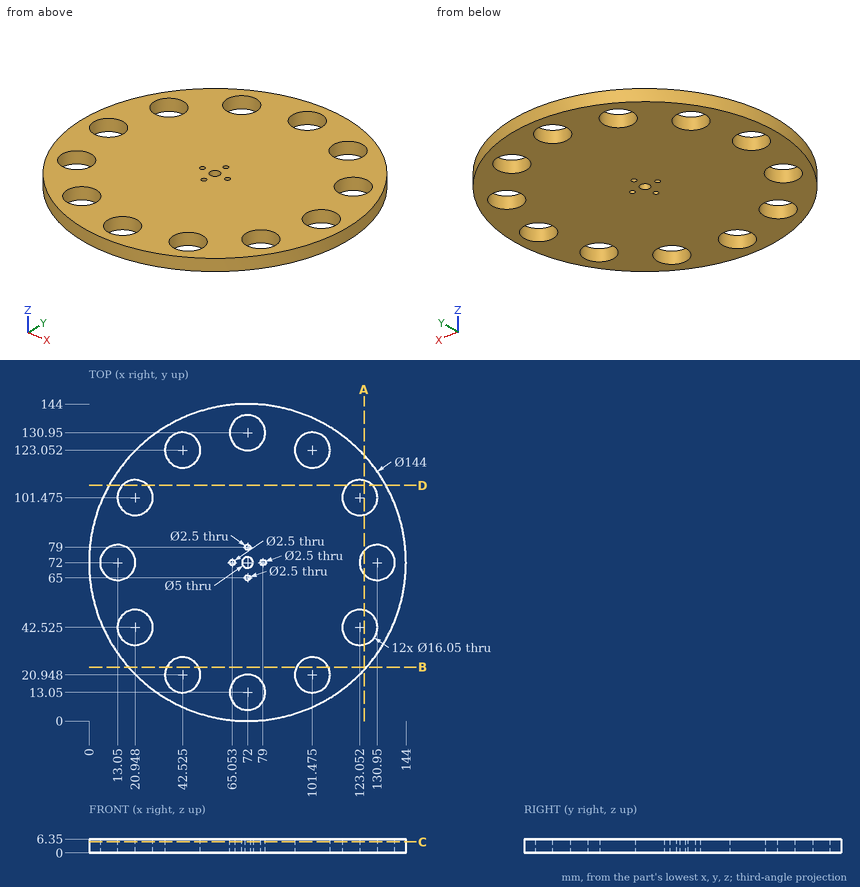
Source: three-view drawing plus pictorial views. Frame: mm from the lowest corner of the part. Round coordinates to 2 decimals unless told otherwise and drop trailing zeros. Loops run counter-clockwise (first coordinate to the right, second up) from the corner with the lowest first, then second, coordinate; pieces in that order, holes last.
1. Ray query, L1, parallel to Y at x = 101, z = 2; L2, parallel to Y at x = 95.5, z = 4.5 (1 decimal); L3, parallel to Y at x = 136, z = 3 (1 decimal). Return the intervals inside material, ascending.
2. Contact query for flat-ended pins moving along their axis: pin 1 (2 mm diameter, centred on x = 65.05, y = 72, fed in from -Z); pin 2 (2 mm diameter, centred on y = 41, z = 3.5, fed in from +X); pin 3 (2 mm diameter, centred on y = 87, z = 2.5, fed in from +X); pin 4 (1 mm diameter, centred on x = 105.5, z = 4.5, fed in from +Y). Output: stop coordinate, or through.
3. Section query D-D on y = 107. Output: boundary loops of the cut face in (x, z), and give its area (3 significant figures).
4. Section query B-B on y = 24.5. Output: boundary loops of the cut face in (x, z).
5. Section query C-C on z = 5. Give the number of separate pieces and of enclosed holes in the cut face, and give its area (3 significant figures).
6. Section query A-A on x = 125. Output: boundary loops of the cut face in (y, z) (3 decimals), and give its area (3 significant figures).
Answers below:
1. L1: y = 6.1 to 12.94, 28.96 to 115.04, 131.06 to 137.9
1. L2: y = 3.9 to 15.6, 26.3 to 117.7, 128.4 to 140.1
1. L3: y = 39 to 65.8, 78.2 to 105
2. pin 1: passes through
2. pin 2: stops at x = 137.45
2. pin 3: stops at x = 142.63
2. pin 4: stops at y = 135.99
3. outline: (9.08, 0) - (15.13, 0) - (15.13, 6.35) - (9.08, 6.35) - close; (26.77, 0) - (117.23, 0) - (117.23, 6.35) - (26.77, 6.35) - close; (128.87, 0) - (134.92, 0) - (134.92, 6.35) - (128.87, 6.35) - close
3. area: 651 mm2
4. outline: (17.89, 0) - (35.33, 0) - (35.33, 6.35) - (17.89, 6.35) - close; (49.72, 0) - (94.28, 0) - (94.28, 6.35) - (49.72, 6.35) - close; (108.67, 0) - (126.11, 0) - (126.11, 6.35) - (108.67, 6.35) - close
5. separate pieces: 1
5. enclosed holes: 17
5. area: 13,800 mm2
6. outline: (23.266, 0) - (34.74, 0) - (34.74, 6.35) - (23.266, 6.35) - close; (50.31, 0) - (66.615, 0) - (66.615, 6.35) - (50.31, 6.35) - close; (77.385, 0) - (93.69, 0) - (93.69, 6.35) - (77.385, 6.35) - close; (109.26, 0) - (120.734, 0) - (120.734, 6.35) - (109.26, 6.35) - close
6. area: 353 mm2
